Design review of the part built by this model. Coordinates are the model's own, in mm. A direction names the side the tool comes from. Round coordinates to 2 decimals unless told otherwise and drop trailing zeros. Loops run counter-clockwise (first coordinate to the right, second up) from the corner with the lowest first, then second, coordinate; pieces in that order, holes last. Notation, with made-up numbers: M -36.75,8.5 L -6.75,8.5 A13 ccw -6.75,28.5 Z; hole C -3,-37.5 d9. An arc over 180 degrees is marked long. One line per item, written item: value. Start each with the question number.
Item 1: For faces 1 (the cylindrical face through (1.507, -3.905, 0.867)), 2 (the cylindrical face through (0.99, 10.49, 0.13)), list the 3-axis set-ups (+Z, -Z, +X, -X, +Y, -Y) from which the entire face can be reached by the end or side of a thin tool; tool diameter is ignored.
Item 2: We need section D-D (y = 9.5). Write out the cut boundary in (x, z).
Item 3: Clearance check with a flat-ended pin moving along its axis: pin 1 (1 mm diameter, centred on x = 2, z = 7, fed in from +Y). State where the tip first meets the part, or that it passes through.
Item 4: We need section A-A (z = 0). State how many separate pieces and enclosed holes the cut face has, then the cut area to 3 significant figures.
Item 5: Mouldability with a two-part tool opening along Y and no side actions: class faces 3 (the cylindrical face through (0.986, 3.755, -11.923)), 4 (the flat face through (2, 3, -1)), 5 (the cylindrical face through (1, -0.6, 10.3)) as released by +Y, released by -Y, zero draft, split by the parting line, or undercut.
Item 6: For line 1 along Z through (x, y) = (1.1, -1.75); line 2 along Y through (x, z) = (1.5, 0); line 3 along Z through (x, y) = (1.5, -0.25), list the stretches that pass through material, from the lowest coordinate up.
from build123d import *

# Parameters (mm, degrees)
SKETCH1_R           = 12.5
SKETCH1_R_2         = 3
SKETCH1_R_3         = 1
BOSS_EXTRUDE1_DEPTH = 2
SKETCH2_R           = 5
SKETCH2_R_2         = 4
CUT_EXTRUDE1_DEPTH  = 1
FILLET1_R           = 1


with BuildPart() as part:
    # Sketch1 → Boss-Extrude1 (new body)
    with BuildSketch(Plane(origin=(0, 0, 0), x_dir=(0, 0, -1), z_dir=(1, 0, 0))):
        Circle(SKETCH1_R)
        Circle(SKETCH1_R_2, mode=Mode.SUBTRACT)
        with Locations((9.5, 0)):
            Circle(SKETCH1_R_3, mode=Mode.SUBTRACT)
        with Locations((6.717514421, -6.717514421)):
            Circle(SKETCH1_R_3, mode=Mode.SUBTRACT)
        with Locations((0, -9.5)):
            Circle(SKETCH1_R_3, mode=Mode.SUBTRACT)
        with Locations((-6.717514421, -6.717514421)):
            Circle(SKETCH1_R_3, mode=Mode.SUBTRACT)
        with Locations((-9.5, 0)):
            Circle(SKETCH1_R_3, mode=Mode.SUBTRACT)
        with Locations((-6.717514421, 6.717514421)):
            Circle(SKETCH1_R_3, mode=Mode.SUBTRACT)
        with Locations((0, 9.5)):
            Circle(SKETCH1_R_3, mode=Mode.SUBTRACT)
        with Locations((6.717514421, 6.717514421)):
            Circle(SKETCH1_R_3, mode=Mode.SUBTRACT)
    extrude(amount=BOSS_EXTRUDE1_DEPTH)

    # Sketch2 → Cut-Extrude1 (cut)
    with BuildSketch(Plane(origin=(2, 0, 0), x_dir=(0, 0, -1), z_dir=(1, 0, 0))):
        Circle(SKETCH2_R)
        Circle(SKETCH2_R_2, mode=Mode.SUBTRACT)
    extrude(amount=-CUT_EXTRUDE1_DEPTH, mode=Mode.SUBTRACT)

    # Fillet1
    fillet1_edges = [part.edges().sort_by_distance(p)[0] for p in [
        (2, 0, 5),
    ]]
    fillet(fillet1_edges, radius=FILLET1_R - 0.0001)  # a hair under: the kernel refuses the full size


solid = part.part
A:
1. face 1: +X
1. face 2: +X, -X
2. outline: M 0,-8.12 L 2,-8.12 L 2,-1 L 0,-1 Z; M 0,1 L 2,1 L 2,8.12 L 0,8.12 Z
3. pin 1: y = 10.68
4. separate pieces: 4
4. enclosed holes: 0
4. area: 27.6 mm2
5. face 3: split by the parting line
5. face 4: zero draft
5. face 5: undercut
6. line 1: -12.38 to -4.69, -3.6 to -2.44, 2.44 to 3.6, 4.69 to 12.38
6. line 2: -12.5 to -10.5, -8.5 to -5.13, -4 to -3, 3 to 4, 5.13 to 8.5, 10.5 to 12.5
6. line 3: -12.5 to -10.47, -8.53 to -5.13, -3.99 to -2.99, 2.99 to 3.99, 5.13 to 8.53, 10.47 to 12.5
